from build123d import *

# Parameters (mm, degrees)
SKETCH_1_W          = 40
SKETCH_1_H          = 30
EXTRUDE_1_DEPTH     = 5
SKETCH_2_W          = 31
SKETCH_2_H          = 28
CUT_EXTRUDE_1_DEPTH = 3.5
CUT_EXTRUDE_2_DEPTH = 26.243811123
EXTRUDE_START       = 8
EXTRUDE_2_DEPTH     = 8
FILLET_START        = 1.5
FILLET_1_DEPTH      = 8.5
CHAMFER_1_SIZE      = 3


with BuildPart() as part:
    # ｽｹｯﾁ1 → ﾎﾞｽ - 押し出し1 (new body)
    with BuildSketch(Plane.XY):
        Rectangle(SKETCH_1_W, SKETCH_1_H)
    extrude(amount=EXTRUDE_1_DEPTH)

    # ｽｹｯﾁ2 → ｶｯﾄ - 押し出し1 (cut)
    with BuildSketch(Plane.XY.offset(5)):
        with Locations((0, -1)):
            Rectangle(SKETCH_2_W, SKETCH_2_H)
    extrude(amount=-CUT_EXTRUDE_1_DEPTH, mode=Mode.SUBTRACT)

    # ｽｹｯﾁ3 → ｶｯﾄ - 押し出し2 (cut, through all)
    with BuildSketch(Plane.XY.offset(1.5)):
        with BuildLine():
            Line((8.5, -2), (8.5, -15))
            Line((8.5, -15), (-8.5, -15))
            Line((-8.5, -15), (-8.5, -2))
            ThreePointArc((-8.5, -2), (0, 6.5), (8.5, -2))
        make_face()
        with BuildLine():
            Line((13, -4.5), (13, 0.5))
            ThreePointArc((13, 0.5), (11.5, 2), (10, 0.5))
            Line((10, 0.5), (10, -4.5))
            ThreePointArc((10, -4.5), (11.5, -6), (13, -4.5))
        make_face()
        with BuildLine():
            Line((-13, -4.5), (-13, 0.5))
            ThreePointArc((-13, 0.5), (-11.5, 2), (-10, 0.5))
            Line((-10, 0.5), (-10, -4.5))
            ThreePointArc((-10, -4.5), (-11.5, -6), (-13, -4.5))
        make_face()
    extrude(amount=-CUT_EXTRUDE_2_DEPTH, mode=Mode.SUBTRACT)

    # ｽｹｯﾁ4 → ﾎﾞｽ - 押し出し2 (add)
    with BuildSketch(Plane.XY.offset(1.5).offset(EXTRUDE_START)):
        with BuildLine():
            Line((-8.5, -2), (-8.5, 13))
            Line((-8.5, 13), (8.5, 13))
            Line((8.5, 13), (8.5, -2))
            ThreePointArc((8.5, -2), (0, 6.5), (-8.5, -2))
        make_face()
    extrude(amount=-EXTRUDE_2_DEPTH)

    # ﾌｨﾚｯﾄ1: read off the stored shape, not the designer's step
    # ﾌｨﾚｯﾄ1 outline → ﾌｨﾚｯﾄ1 (cut)
    with BuildSketch(Plane.XY.offset(FILLET_START)):
        with BuildLine():
            ThreePointArc((8.5, 2.123105626), (8.117851131, 1.637192968), (7.555555556, 1.894044202))
            ThreePointArc((7.555555556, 1.894044202), (8.260515184, 0.003469213), (8.5, -2))
            Line((8.5, -2), (8.5, 2.123105626))
        make_face()
        with BuildLine():
            ThreePointArc((-7.555555556, 1.894044202), (-8.117851131, 1.637192968), (-8.5, 2.123105626))
            Line((-8.5, 2.123105626), (-8.5, -2))
            ThreePointArc((-8.5, -2), (-8.260515184, 0.003469213), (-7.555555556, 1.894044202))
        make_face()
    extrude(amount=FILLET_1_DEPTH, mode=Mode.SUBTRACT)

    # 面取り1
    chamfer_1_edges = [part.edges().sort_by_distance(p)[0] for p in [
        (0, 13, 9.5),
    ]]
    chamfer(chamfer_1_edges, length=CHAMFER_1_SIZE)


solid = part.part
Geometry check sheet. Reference: the model listing, model coordinates, mm. A direction names the side the tool comes from. Give positions to 0.01 mm unless a question says otherwise; leave off trailing zeros. Write each loop counter-clockwise with the first axis right and the second up, starting at its lowest first coordinate (ties: lowest second). Pieces come first, ordered by that corner, then holes.
1) Cross-section at A-A (x = 11.5). Record the boundary of the cut face in (y, z).
Values follow:
outline: (-15, 0) - (-6, 0) - (-6, 1.5) - (-15, 1.5) - close; (2, 0) - (15, 0) - (15, 5) - (13, 5) - (13, 1.5) - (2, 1.5) - close
2) Thickness scan on line 1 (X direction, y = 10.75, z = 3.5); line 2 (X direction, y = -1.75, z = 2.5); line 3 (X direction, y = 10, z = 6). Record the ranges inside material, lowest first.
Values follow:
line 1: x = -20 to -15.5, -8.5 to 8.5, 15.5 to 20
line 2: x = -20 to -15.5, 15.5 to 20
line 3: x = -8.5 to 8.5
3) Release check for a two-part mould opening along Y. For faces 1 (the face through (-0.1, 11.5, 8)), 2 (the face through (13.2, -0.8, 1.5)), 3 (the face through (-13, -2, 1)) record: released by +Y, released by -Y, zero draft, split by the parting line, or undercut.
Values follow:
face 1: released by +Y
face 2: zero draft
face 3: undercut
4) Cross-section at D-D (y = 8.75). Record the boundary of the cut face in (x, z).
Values follow:
outline: (-20, 0) - (20, 0) - (20, 5) - (15.5, 5) - (15.5, 1.5) - (8.5, 1.5) - (8.5, 9.5) - (-8.5, 9.5) - (-8.5, 1.5) - (-15.5, 1.5) - (-15.5, 5) - (-20, 5) - close
5) Set-up check for faces 4 (the face through (15.5, -1, 3)), 5 (the face through (-10, -2, 1)), 6 (the face through (8.5, -8, 1)): record each of +Z, -Z, +X, -X, +Y, -Y from which the full face is reachable in a straight line by a thin tool's end or side.
Values follow:
face 4: +Z, -Y
face 5: +Z, -Z
face 6: +Z, -Z, -Y
6) Cross-section at B-B (y = -11). Record the boundary of the cut face in (x, z), plus the area to 3 significant figures.
Values follow:
outline: (-20, 0) - (-8.5, 0) - (-8.5, 1.5) - (-15.5, 1.5) - (-15.5, 5) - (-20, 5) - close; (8.5, 0) - (20, 0) - (20, 5) - (15.5, 5) - (15.5, 1.5) - (8.5, 1.5) - close
area: 66.0 mm2
7) Cross-section at C-C (x = 0). Record the boundary of the cut face in (y, z), plus the area to 4 significant figures.
Values follow:
outline: (6.5, 0) - (15, 0) - (15, 5) - (13, 5) - (13, 6.5) - (10, 9.5) - (6.5, 9.5) - close
area: 67.25 mm2
8) Go/stop test with a flat-tipped pin: pin 1 Ø8.5 at (x, y) = (-13, -2) entering from +Z. Record where the tip stops, or that it passes through.
Values follow:
pin 1: stops at z = 5
